CAD build for the part. Positions are in the model's coordinates, mm. Coordinates: 2 decimals unless noted, no trailing zeros. Loops run counter-clockwise (first coordinate to the right, second up) from the corner with the lowest first, then second, coordinate; pieces in that order, holes last. Notation, with made-up numbers: M 32,42 L 39,42 A11 cw 39,55 Z; hole C 54,18.5 d4. An arc over 180 degrees is marked long. Answer as a JSON object with one key per item and string values. Group by question number.
```python
from build123d import *

# Parameters (mm, degrees)
SKETCH1_W           = 357.50000001
SKETCH1_H           = 570
BOSS_EXTRUDE1_DEPTH = 18
SKETCH5_W           = 18
SKETCH5_H           = 557.3
CUT_EXTRUDE3_DEPTH  = 6.35
SKETCH7_W           = 357.50000001
SKETCH7_H           = 18
CUT_EXTRUDE4_DEPTH  = 6.35
FILLET1_R           = 9.525


with BuildPart() as part:
    # Sketch1 → Boss-Extrude1 (new body)
    with BuildSketch(Plane(origin=(0, 0, 0), x_dir=(0, 0, -1), z_dir=(1, 0, 0))):
        with Locations((178.750000005, 285)):
            Rectangle(SKETCH1_W, SKETCH1_H)
    extrude(amount=BOSS_EXTRUDE1_DEPTH)

    # Sketch5 → Cut-Extrude3 (cut)
    with BuildSketch(Plane(origin=(18, 0, 0), x_dir=(0, 0, -1), z_dir=(1, 0, 0))):
        with Locations((47.1, 285)):
            Rectangle(SKETCH5_W, SKETCH5_H)
    extrude(amount=-CUT_EXTRUDE3_DEPTH, mode=Mode.SUBTRACT)

    # Sketch7 → Cut-Extrude4 (cut)
    with BuildSketch(Plane(origin=(18, 0, 0), x_dir=(0, 0, -1), z_dir=(1, 0, 0))):
        with Locations((178.750000005, 9)):
            Rectangle(SKETCH7_W, SKETCH7_H)
        with Locations((178.750000005, 561)):
            Rectangle(SKETCH7_W, SKETCH7_H)
    extrude(amount=-CUT_EXTRUDE4_DEPTH, mode=Mode.SUBTRACT)

    # Fillet1
    fillet1_edges = [part.edges().sort_by_distance(p)[0] for p in [
        (5.825, 0, 0),
        (0, 570, -178.750000005),
        (0, 0, -178.750000005),
        (5.825, 570, 0),
        (0, 285, 0),
    ]]
    fillet(fillet1_edges, radius=FILLET1_R)


solid = part.part
```
Item 1: Slice it at A-A, the plane z = -132.5. Write the cut outline in (x, y) (3 decimals), then the cut area to 3 significant figures.
Item 2: Slice it at B-B, the plane y = 447. Write the cut outline in (x, z) (3 decimals), then the cut area to 3 significant figures.
Item 3: Drill centre lines: L1, parallel to Z at x = 12.5, y = 103; L2, parallel to Y at x = 14.5, z = -36; L3, parallel to Z at x = 8, y = 26. Where is each one in solid material? Low to high. Write a range as from..to.
Item 4: Pin check, flat tips, straight feed: pin 1 (1.9 mm diameter, centred on x = 14.5, z = -223.5, fed in from -Y); pin 2 (8 mm diameter, centred on x = 6, z = -244.5, fed in from -Y); pin 3 (6 mm diameter, centred on x = 15.5, z = -83, fed in from +Y); pin 4 (2 mm diameter, centred on x = 7.5, z = -56.5, fed in from -Y). Stop position of each tip, or through.
Item 5: Pull direction Z, two halves, no side cores. Call faces 1 (the flat face through (9, 281, -357.5)), 2 (the flat face through (11.65, 286, -46)), 3 (the flat face through (18, 289, -19)): released by +Z, released by -Z, zero draft, split by the parting line, or undercut.
Computed:
{
 "1": {"outline": "M 0,9.525 A9.525 ccw 9.525,0 L 11.65,0 L 11.65,18 L 18,18 L 18,552 L 11.65,552 L 11.65,570 L 9.525,570 A9.525 ccw 0,560.475 Z", "area": "9,990 mm2"},
 "2": {"outline": "M 0,-357.5 L 18,-357.5 L 18,-56.1 L 11.65,-56.1 L 11.65,-38.1 L 18,-38.1 L 18,0 L 9.525,0 A9.525 ccw 0,-9.525 Z", "area": "6,300 mm2"},
 "3": {"L1": "-357.5..-56.1, -38.1..0", "L2": "18..552", "L3": "-357.5..-0.12"},
 "4": {"pin 1": "y = 18", "pin 2": "y = 0", "pin 3": "y = 552", "pin 4": "y = 0.06"},
 "5": {"face 1": "released by -Z", "face 2": "undercut", "face 3": "zero draft"}
}
